Part model, mm, in its own coordinate system. Coordinates: 2 decimals unless noted, no trailing zeros. Loops run counter-clockwise (first coordinate to the right, second up) from the corner with the lowest first, then second, coordinate; pieces in that order, holes last. Notation, with made-up numbers: (73, 23.25) - (123, 23.25) arc R33 cw to (123, 52.25) - close; hole circle Ø4 at (53.25, 82). An arc over 180 degrees is marked (long way). One line per question, with ' | ' between items. Start each with the question number.
Autodesk Inventor part; units mm, degrees
ref_plane "Start Plane" through (0, 0, 20) normal (0, 0, 1) x (1, 0, 0)
ref_plane "End Plane" through (0, 0, 1980) normal (0, 0, 1) x (1, 0, 0)
ref_plane "Work Plane4" through (1200, -15.5, 1980) normal (0, 0, 1) x (1, 0, 0)
ref_plane "Start Plane" through (0, 0, 20) normal (0, 0, 1) x (1, 0, 0)
ref_plane "End Plane" through (0, 0, 1980) normal (0, 0, 1) x (1, 0, 0)
sketch "Sketch" plane through (0, 0, 0) normal (0, 0, 1) x (1, 0, 0)
  line L0 (-20, -15.5) -> (-20, 15.5)
  line L1 (-15.5, 20) -> (15.5, 20)
  line L2 (20, 15.5) -> (20, -15.5)
  line L3 (15.5, -20) -> (-15.5, -20)
  arc A0 (-20, -15.5) -> (-15.5, -20) centre (-15.5, -15.5) ccw
  arc A1 (-15.5, 20) -> (-20, 15.5) centre (-15.5, 15.5) ccw
  arc A2 (20, 15.5) -> (15.5, 20) centre (15.5, 15.5) ccw
  arc A3 (15.5, -20) -> (20, -15.5) centre (15.5, -15.5) ccw
  arc A4 (-15.5, 17) -> (-17, 15.5) centre (-15.5, 15.5) ccw
  line L4 (-15.5, 17) -> (15.5, 17)
  arc A5 (17, 15.5) -> (15.5, 17) centre (15.5, 15.5) ccw
  line L5 (17, 15.5) -> (17, -15.5)
  arc A6 (15.5, -17) -> (17, -15.5) centre (15.5, -15.5) ccw
  line L6 (15.5, -17) -> (-15.5, -17)
  arc A7 (-17, -15.5) -> (-15.5, -17) centre (-15.5, -15.5) ccw
  line L7 (-17, -15.5) -> (-17, 15.5)
  line L8 (0, 29.3048) -> (0, -29.3048) construction
  line L9 (-29.3048, 0) -> (29.3048, 0) construction
  dimension "d7" = 4.5
  dimension "d10" = 40
  dimension "d11" = 40
  dimension "d12" = 3
  dimension "d15" = 20
  dimension "d16" = 20
extrude "Body" add sketch "Sketch" along normal up to surface (1960 mm away) from surface at 20
sketch "Sketch3" plane through (0, 0, 0) normal (0, 0, 1) x (1, 0, 0)
  line L0 (0, 0) -> (10, 0)
ref_plane "Work Plane3" through (0, 0, 0) normal (0, -1, 0) x (1, 0, 0)
ref_plane "Work Plane4" through (1200, -15.5, 1980) normal (0, 0, 1) x (1, 0, 0)
split "Split1" plane through (1200, -15.5, 1980) removes the side toward (0, 0, 1)
ref_plane "Work Plane5" through (0, -15.5, 20) normal (0, 0, -1) x (-1, 0, 0)
split "Split2" plane through (0, -15.5, 20) removes the side toward (0, 0, -1)
sketch "Sketch4" plane through (0, 0, 0) normal (0, -1, 0) x (1, 0, 0)
  line L0 (-2, 20) -> (12, 20)
  line L1 (-2, 1980) -> (12, 1980)
  dimension "d18" = 1960
equation "\"d7\" = G_IR"
equation "\"d10\" = G_H"
equation "\"d11\" = G_W"
equation "\"d12\" = G_T"
equation "\"d15\" = 0.5 * d10"
equation "\"d16\" = 0.5 * d11"
equation "\"d3\" = G_L"
equation "\"G_W\" = 40"
equation "\"G_H\" = 40"
equation "\"G_T\" = 3"
equation "\"G_IR\" = 4.5"
equation "\"G_L\" = d18"
properties part number "ISO 12633-2 - 40x40x3 - 1960" material "Steel, Mild"
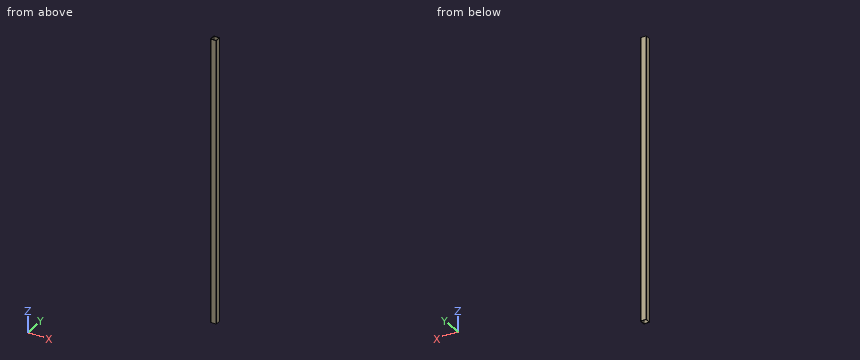
1) Pin check, flat tip, straight feed: pin 1 Ø10 at (x, y) = (-10.5, 11) entering from -Z. Stop position of the tip, or through.
2) Wall check: line 1 along X through (y, z) = (16, 1582.5); line 2 along X through (y, z) = (9.5, 1711). Give the ranges that are in metal, low to high. Write a range as [from, to].
3) Band-saw the part on B-B on y = 8.5. List the corners of the cut face in (x, z).
4) Band-saw the part on A-A on z = 1595. List the corners of the cut face in (x, y), then the cut area to 3 significant figures.
Values found:
1) pin 1: through
2) line 1: [-19.97, -16.91], [16.91, 19.97] | line 2: [-20, -17], [17, 20]
3) outline: (-20, 20) - (-17, 20) - (-17, 1980) - (-20, 1980) - close; (17, 20) - (20, 20) - (20, 1980) - (17, 1980) - close
4) outline: (-20, -15.5) arc R4.5 ccw to (-15.5, -20) - (15.5, -20) arc R4.5 ccw to (20, -15.5) - (20, 15.5) arc R4.5 ccw to (15.5, 20) - (-15.5, 20) arc R4.5 ccw to (-20, 15.5) - close; hole (-17, -15.5) arc R1.5 ccw to (-15.5, -17) - (15.5, -17) arc R1.5 ccw to (17, -15.5) - (17, 15.5) arc R1.5 ccw to (15.5, 17) - (-15.5, 17) arc R1.5 ccw to (-17, 15.5) - close | area: 429 mm²
